Can you work these out from the model? Positions are in its coordinate system, mm. Coordinates: 2 decimals unless noted, no trailing zeros. Order: outer loops, then holes, each group sorted by start corner. A loop starts at its lowest first (then second) coordinate and runs counter-clockwise, first axis right, second up. Notation, with made-up numbers: M 11,66.5 L 51,66.5 A14 cw 51,75.5 Z; hole C 60.5,-19.5 d7. An arc over 180 degrees is marked long. Answer as CSV lines item,"result". Start each with the question number.
1. If we section it at B-B (y = -35): List the corners of the cut face in (x, z) for me, plus the area to 3 significant figures.
2. If we mould it in two halves opening along Y, with no side actions, what happens to faces 1 (the face through (-1, -42.5, 2)), 2 (the face through (-42.5, -1, 2)), 3 (the face through (-35.267, 37.033, 1.521)), 4 (the face through (24.67, -22.52, 1.52))? For each: released by +Y, released by -Y, zero draft, split by the parting line, or undercut.
3. If we section it at C-C (z = 1.7): Give the number of separate pieces and of enclosed holes in the cut face, plus the area to 3 significant figures.
4. If we section it at A-A (x = 25): List the corners of the cut face in (y, z) for me, plus the area to 3 significant figures.
5. I need wall thicknesses on line 1 along Y through (x, z) = (-25, 0.85); line 2 along X through (y, z) = (-33.5, 0.5); line 3 along Y through (x, z) = (35, 0.85). Which ranges of each line are inside material? Lowest first, please. Write a range as from..to.
```python
from build123d import *

# Parameters (mm, degrees)
SKETCH1_W           = 65
SKETCH1_H           = 65
SKETCH1_R           = 2.55
BOSS_EXTRUDE1_DEPTH = 3
SKETCH2_W           = 85
SKETCH2_H           = 85
SKETCH2_R           = 2.05
SKETCH2_R_2         = 2.5
BOSS_EXTRUDE2_DEPTH = 3


with BuildPart() as part:
    # Sketch1 → Boss-Extrude1 (new body)
    with BuildSketch(Plane.XY):
        Rectangle(SKETCH1_W, SKETCH1_H)
        with Locations((-25, 25)):
            Circle(SKETCH1_R, mode=Mode.SUBTRACT)
        with Locations((25, 25)):
            Circle(SKETCH1_R, mode=Mode.SUBTRACT)
        with Locations((-25, -25)):
            Circle(SKETCH1_R, mode=Mode.SUBTRACT)
        with Locations((25, -25)):
            Circle(SKETCH1_R, mode=Mode.SUBTRACT)
    extrude(amount=BOSS_EXTRUDE1_DEPTH)

    # Sketch2 → Boss-Extrude2 (add)
    with BuildSketch(Plane.XY.offset(3)):
        Rectangle(SKETCH2_W, SKETCH2_H)
        with Locations((-35, 35)):
            Circle(SKETCH2_R, mode=Mode.SUBTRACT)
        with Locations(Location((35, 35, 0), (0, 0, 180))):
            Circle(SKETCH2_R, mode=Mode.SUBTRACT)
        with Locations((35, -35)):
            Circle(SKETCH2_R, mode=Mode.SUBTRACT)
        with Locations(Location((-35, -35, 0), (0, 0, 180))):
            Circle(SKETCH2_R, mode=Mode.SUBTRACT)
        with Locations((-25, 25)):
            Circle(SKETCH2_R_2, mode=Mode.SUBTRACT)
        with Locations((25, 25)):
            Circle(SKETCH2_R_2, mode=Mode.SUBTRACT)
        with Locations((25, -25)):
            Circle(SKETCH2_R_2, mode=Mode.SUBTRACT)
        with Locations((-25, -25)):
            Circle(SKETCH2_R_2, mode=Mode.SUBTRACT)
    extrude(amount=-BOSS_EXTRUDE2_DEPTH)


solid = part.part
```
Solved:
1,outline,"M -42.5,0 L -37.05,0 L -37.05,3 L -42.5,3 Z; M -32.95,0 L 32.95,0 L 32.95,3 L -32.95,3 Z; M 37.05,0 L 42.5,0 L 42.5,3 L 37.05,3 Z"
1,area,"230 mm²"
2,face 1,"released by -Y"
2,face 2,"zero draft"
2,face 3,"undercut"
2,face 4,"undercut"
3,separate pieces,"1"
3,enclosed holes,"8"
3,area,"7,090 mm²"
4,outline,"M -42.5,0 L -27.5,0 L -27.5,3 L -42.5,3 Z; M -22.5,0 L 22.5,0 L 22.5,3 L -22.5,3 Z; M 27.5,0 L 42.5,0 L 42.5,3 L 27.5,3 Z"
4,area,"225 mm²"
5,line 1,"-42.5..-27.5, -22.5..22.5, 27.5..42.5"
5,line 2,"-42.5..-36.4, -33.6..33.6, 36.4..42.5"
5,line 3,"-42.5..-37.05, -32.95..32.95, 37.05..42.5"
